The listing builds one solid part. Answer for the finished solid, in the listing's coordinates (mm). A direction names the side the tool comes from. Give positions to 0.01 mm unless a question says otherwise; leave off trailing zeros. Order: outer loops, then holes, each group sorted by start corner. A loop starts at its lowest first (then second) coordinate and runs counter-clockwise, first axis right, second up.
```python
from build123d import *

# Parameters (mm, degrees)
SKETCH_1_R               = 34.4
SKETCH_1_R_2             = 31.4
EXTRUDE_1_DEPTH          = 5.4
SKETCH_2_R               = 35.4
SKETCH_2_R_2             = 30.4
EXTRUDE_1_2_DEPTH        = 4
SKETCH_3_R               = 0.5
CUT_EXTRUDE_1_DEPTH      = 3
PATTERN_CIRCULAR_1_COUNT = 6
SKETCH_4_OUTSIDE_W       = 92.914
SKETCH_4_OUTSIDE_H       = 92.914
SKETCH_4_OUTSIDE_R       = 34.3
SKETCH_4_OUTSIDE_R_2     = 31.5
CUT_EXTRUDE_2_DEPTH      = 5.4
SKETCH_5_OUTSIDE_W       = 92.914
SKETCH_5_OUTSIDE_H       = 92.914
SKETCH_5_OUTSIDE_R       = 35.3
SKETCH_5_OUTSIDE_R_2     = 30.5
CUT_EXTRUDE_3_DEPTH      = 51.938001531


with BuildPart() as part:
    # 草图1 → Extrude 1 (new body)
    with BuildSketch(Plane(origin=(0, 0, 0), x_dir=(1, 0, 0), z_dir=(0, 1, 0))):
        Circle(SKETCH_1_R)
        Circle(SKETCH_1_R_2, mode=Mode.SUBTRACT)
    extrude(amount=EXTRUDE_1_DEPTH)

    # 草图2 → Extrude 1 2 (add)
    with BuildSketch(Plane(origin=(0, 5.4, 0), x_dir=(1, 0, 0), z_dir=(0, 1, 0))):
        with Locations(Location((0, 0, 0), (0, 0, 270))):
            Circle(SKETCH_2_R)
        with Locations(Location((0, 0, 0), (0, 0, 270))):
            Circle(SKETCH_2_R_2, mode=Mode.SUBTRACT)
    extrude(amount=EXTRUDE_1_2_DEPTH)

    # 草图3 → 切除-拉伸1 (cut)
    with BuildSketch(Plane.XZ):
        with Locations(Location((0, 32.9, 0), (0, 0, 270))):
            Circle(SKETCH_3_R)
    cut_extrude_1 = extrude(amount=-CUT_EXTRUDE_1_DEPTH, mode=Mode.SUBTRACT)

    # 阵列(圆周)1: 切除-拉伸1 ×6 about axis
    pattern_circular_1_axis = Axis((0, 0, 0), (0, 1, 0))
    for i in range(1, PATTERN_CIRCULAR_1_COUNT):
        add(cut_extrude_1.rotate(pattern_circular_1_axis, i * 360 / PATTERN_CIRCULAR_1_COUNT), mode=Mode.SUBTRACT)

    # 草图4 outside → 切除-拉伸2 (cut)
    # profile 1 of 2: a face of its own
    with BuildSketch(Plane.XZ):
        Rectangle(SKETCH_4_OUTSIDE_W, SKETCH_4_OUTSIDE_H)
        with Locations(Location((0, 0, 0), (0, 0, 270))):
            Circle(SKETCH_4_OUTSIDE_R, mode=Mode.SUBTRACT)
    # profile 2 of 2: a face of its own
    with BuildSketch(Plane.XZ):
        with Locations(Location((0, 0, 0), (0, 0, 270))):
            Circle(SKETCH_4_OUTSIDE_R_2)
    extrude(amount=-CUT_EXTRUDE_2_DEPTH, mode=Mode.SUBTRACT)

    # 草图5 outside → 切除-拉伸3 (cut, through all)
    # profile 1 of 2: a face of its own
    with BuildSketch(Plane.XZ):
        Rectangle(SKETCH_5_OUTSIDE_W, SKETCH_5_OUTSIDE_H)
        with Locations(Location((0, 0, 0), (0, 0, 270))):
            Circle(SKETCH_5_OUTSIDE_R, mode=Mode.SUBTRACT)
    # profile 2 of 2: a face of its own
    with BuildSketch(Plane.XZ):
        with Locations(Location((0, 0, 0), (0, 0, 270))):
            Circle(SKETCH_5_OUTSIDE_R_2)
    extrude(amount=-CUT_EXTRUDE_3_DEPTH, mode=Mode.SUBTRACT)


solid = part.part
```
1) Straight lines are drawn through the part: probe 1 along X at (y, z) = (4, 0); probe 2 along X at (y, z) = (9, -1); probe 3 along X at (y, z) = (2.35, -16.45). For each, find the intervals that lie inside material, in ascending order.
Geometry says:
probe 1: x = -34.3 to -31.5, 31.5 to 34.3
probe 2: x = -35.29 to -30.48, 30.48 to 35.29
probe 3: x = -30.1 to -28.99, -27.99 to -26.86, 26.86 to 27.99, 28.99 to 30.1
2) For a pull along X with two mould halves and no side action, classify faces 3 (the cylindrical face through (10.303, 2.662, -32.716)), 4 (the cylindrical face through (-29.775, 7.372, 6.612)), 5 (the flat face through (15, 0, 28)) as +X half, -X half, draft (parallel to the pull), parting line (faces both ways), or undercut.
Geometry says:
face 3: parting line
face 4: undercut
face 5: draft
3) Find section A-A (z = 19.5). Write down the section's boundary in (x, y), then the cut area to 3 significant figures.
Geometry says:
outline: (-29.43, 5.4) - (-28.22, 5.4) - (-28.22, 0) - (-24.74, 0) - (-24.74, 5.4) - (-23.45, 5.4) - (-23.45, 9.4) - (-29.43, 9.4) - close; (23.45, 5.4) - (24.74, 5.4) - (24.74, 0) - (28.22, 0) - (28.22, 5.4) - (29.43, 5.4) - (29.43, 9.4) - (23.45, 9.4) - close
area: 85.4 mm2
4) Given P1, Ø0.8, axis at x = 28.5, z = -16.5, coming from the -Y side; P2, Ø5, axis at y = 8, z = -9.5, coming from the -X side; P3, Ø2, axis at x = 23.5, y = 3.5, coming from the +Z side; P4, Ø21, axis at x = -2, z = -16, coming from the -Y side, each flat-ended and moving along its own axis, determine where each tip first touches the part or whether it passes through.
Geometry says:
P1: stops at y = 3
P2: stops at x = -34.6
P3: stops at z = 25.89
P4: passes through
5) Find section C-C (y = 6.25). Write down the section's boundary in (x, z).
Geometry says:
outline: circle Ø70.6 at (0, 0); hole circle Ø61 at (0, 0)
6) Find section B-B (x = 13). Write down the section's boundary in (y, z).
Geometry says:
outline: (0, -31.74) - (5.4, -31.74) - (5.4, -32.82) - (9.4, -32.82) - (9.4, -27.59) - (5.4, -27.59) - (5.4, -28.69) - (0, -28.69) - close; (0, 28.69) - (5.4, 28.69) - (5.4, 27.59) - (9.4, 27.59) - (9.4, 32.82) - (5.4, 32.82) - (5.4, 31.74) - (0, 31.74) - close
7) A tool of negligible diameter and unlimited length cuts with its end or side. For faces 1 (the cylindrical face through (31.232, 2.662, 4.101)), 2 (the cylindrical face through (-21.48, 7.37, 28.01)), from which of +Z, -Z, +X, -X, +Y, -Y can it reach the whole face along a straight path? Write none if from no direction.
Geometry says:
face 1: -Y
face 2: +Y, -Y
